Geometry: final body of the model. Coordinates: model frame, mm. Face numbers are marked on the shaded views. A direction names the side the tool comes from. Give positions to 0.01 mm unless a question says otherwise; leave off trailing zeros. Write each loop counter-clockwise with the first axis right and the second up, starting at its lowest first coordinate (ties: lowest second). Pieces come first, ordered by that corner, then holes. Notation, with made-up numbers: (83, 21) - (125, 21) arc R21 cw to (125, 57) - close; hole circle Ø1 at (-34.5, -21). An arc over 180 degrees is marked (long way). Return JSON: item names as keys, results as strings.
from build123d import *

# Parameters (mm, degrees)
SKETCH1_W           = 150
SKETCH1_H           = 150
BASE_FLANGE1_DEPTH  = 7
SKETCH23_W          = 150
SKETCH23_H          = 150
SKETCH23_W_2        = 130
SKETCH23_H_2        = 130
BOSS_EXTRUDE3_DEPTH = 20
SKETCH27_W          = 7
SKETCH27_H          = 150
BOSS_EXTRUDE4_DEPTH = 20
SKETCH28_W          = 150
SKETCH28_H          = 7
BOSS_EXTRUDE5_DEPTH = 20
SKETCH29_W          = 7
SKETCH29_H          = 150
BOSS_EXTRUDE6_DEPTH = 20
SKETCH30_W          = 150
SKETCH30_H          = 7
BOSS_EXTRUDE7_DEPTH = 20
SKETCH31_R          = 2.5
CUT_EXTRUDE1_DEPTH  = 20
SKETCH32_R          = 2.5
CUT_EXTRUDE2_DEPTH  = 20
FILLET1_R           = 5


# Sheet-metal steps are written as plain solids
with BuildPart() as part:
    # Sketch1 → Base-Flange1 (new body)
    with BuildSketch(Plane.XY):
        Rectangle(SKETCH1_W, SKETCH1_H)
    extrude(amount=-BASE_FLANGE1_DEPTH)

    # Sketch23 → Boss-Extrude3 (add)
    with BuildSketch(Plane(origin=(0, 0, -7), x_dir=(-1, 0, 0), z_dir=(0, 0, -1))):
        Rectangle(SKETCH23_W, SKETCH23_H)
        Rectangle(SKETCH23_W_2, SKETCH23_H_2, mode=Mode.SUBTRACT)
    extrude(amount=BOSS_EXTRUDE3_DEPTH)

    # Sketch27 → Boss-Extrude4 (add)
    with BuildSketch(Plane(origin=(75, 0, 0), x_dir=(0, 0, -1), z_dir=(1, 0, 0))):
        with Locations((23.5, 0)):
            Rectangle(SKETCH27_W, SKETCH27_H)
    extrude(amount=BOSS_EXTRUDE4_DEPTH)

    # Sketch28 → Boss-Extrude5 (add)
    with BuildSketch(Plane(origin=(0, -75, 0), x_dir=(-1, 0, 0), z_dir=(0, -1, 0))):
        with Locations((0, 23.5)):
            Rectangle(SKETCH28_W, SKETCH28_H)
    extrude(amount=BOSS_EXTRUDE5_DEPTH)

    # Sketch29 → Boss-Extrude6 (add)
    with BuildSketch(Plane.ZY.offset(75)):
        with Locations((-23.5, 0)):
            Rectangle(SKETCH29_W, SKETCH29_H)
    extrude(amount=BOSS_EXTRUDE6_DEPTH)

    # Sketch30 → Boss-Extrude7 (add)
    with BuildSketch(Plane(origin=(0, 75, 0), x_dir=(1, 0, 0), z_dir=(0, 1, 0))):
        with Locations((0, 23.5)):
            Rectangle(SKETCH30_W, SKETCH30_H)
    extrude(amount=BOSS_EXTRUDE7_DEPTH)

    # Sketch31 → Cut-Extrude1 (cut)
    with BuildSketch(Plane.XY):
        with Locations((-50, -50)):
            Circle(SKETCH31_R)
        with Locations((-50, 50)):
            Circle(SKETCH31_R)
        with Locations((50, 50)):
            Circle(SKETCH31_R)
        with Locations((50, -50)):
            Circle(SKETCH31_R)
        with Locations((37.5, 37.5)):
            Circle(SKETCH31_R)
        with Locations((-37.5, 37.5)):
            Circle(SKETCH31_R)
        with Locations((37.5, -37.5)):
            Circle(SKETCH31_R)
        with Locations((-37.5, -37.5)):
            Circle(SKETCH31_R)
    extrude(amount=-CUT_EXTRUDE1_DEPTH, mode=Mode.SUBTRACT)

    # Sketch32 → Cut-Extrude2 (cut)
    with BuildSketch(Plane.XY.offset(-20)):
        with Locations((85, 55)):
            Circle(SKETCH32_R)
        with Locations((85, -55)):
            Circle(SKETCH32_R)
        with Locations((55, -85)):
            Circle(SKETCH32_R)
        with Locations((-55, -85)):
            Circle(SKETCH32_R)
        with Locations((-85, -55)):
            Circle(SKETCH32_R)
        with Locations((-85, 55)):
            Circle(SKETCH32_R)
        with Locations((-55, 85)):
            Circle(SKETCH32_R)
        with Locations((55, 85)):
            Circle(SKETCH32_R)
    extrude(amount=-CUT_EXTRUDE2_DEPTH, mode=Mode.SUBTRACT)

    # Fillet1
    # the kernel refuses this fillet: 5 mm, written as the material it takes off along each edge
    with BuildSketch(Plane(origin=(70, -70, -5), x_dir=(0, 0, 1), z_dir=(0, -1, 0))) as fillet1_piece_1_section:
        Polygon((0, 0), (FILLET1_R, 0), (FILLET1_R, -FILLET1_R), (0, -FILLET1_R), align=None)
    fillet1_piece_1 = extrude(amount=FILLET1_R, mode=Mode.PRIVATE)
    fillet1_piece_1 = fillet1_piece_1 - Plane(origin=(70, -70, -5), x_dir=(-0.7071067811865475, 0, -0.7071067811865475), z_dir=(0, -1, 0)) * Sphere(FILLET1_R, mode=Mode.PRIVATE)
    add(fillet1_piece_1, mode=Mode.SUBTRACT)
    with BuildSketch(Plane(origin=(70, 70, -5), x_dir=(1, 0, 0), z_dir=(0, 0, 1))) as fillet1_piece_2_section:
        Polygon((0, 0), (FILLET1_R, 0), (FILLET1_R, FILLET1_R), (0, FILLET1_R), align=None)
    fillet1_piece_2 = extrude(amount=FILLET1_R, mode=Mode.PRIVATE)
    fillet1_piece_2 = fillet1_piece_2 - Plane(origin=(70, 70, -5), x_dir=(-0.7071067811865475, -0.7071067811865475, 0), z_dir=(0, 0, 1)) * Sphere(FILLET1_R, mode=Mode.PRIVATE)
    add(fillet1_piece_2, mode=Mode.SUBTRACT)
    with BuildSketch(Plane(origin=(-70, -70, -5), x_dir=(0, 0, 1), z_dir=(0, -1, 0))) as fillet1_piece_3_section:
        Polygon((0, 0), (FILLET1_R, 0), (FILLET1_R, FILLET1_R), (0, FILLET1_R), align=None)
    fillet1_piece_3 = extrude(amount=FILLET1_R, mode=Mode.PRIVATE)
    fillet1_piece_3 = fillet1_piece_3 - Plane(origin=(-70, -70, -5), x_dir=(0.7071067811865475, 0, -0.7071067811865475), z_dir=(0, -1, 0)) * Sphere(FILLET1_R, mode=Mode.PRIVATE)
    add(fillet1_piece_3, mode=Mode.SUBTRACT)
    with BuildSketch(Plane(origin=(-70, 70, -5), x_dir=(-1, 0, 0), z_dir=(0, 0, 1))) as fillet1_piece_4_section:
        Polygon((0, 0), (FILLET1_R, 0), (FILLET1_R, -FILLET1_R), (0, -FILLET1_R), align=None)
    fillet1_piece_4 = extrude(amount=FILLET1_R, mode=Mode.PRIVATE)
    fillet1_piece_4 = fillet1_piece_4 - Plane(origin=(-70, 70, -5), x_dir=(0.7071067811865475, -0.7071067811865475, 0), z_dir=(0, 0, 1)) * Sphere(FILLET1_R, mode=Mode.PRIVATE)
    add(fillet1_piece_4, mode=Mode.SUBTRACT)
    with BuildSketch(Plane(origin=(75, -75, -20), x_dir=(-1, 0, 0), z_dir=(0, 0, 1)), Plane(origin=(75, 75, -20), x_dir=(0, -1, 0), z_dir=(0, 0, 1)), Plane(origin=(-75, -75, -5), x_dir=(1, 0, 0), z_dir=(0, 0, -1)), Plane(origin=(-75, 75, -5), x_dir=(0, -1, 0), z_dir=(0, 0, -1))) as fillet1_piece_5:
        with BuildLine():
            CenterArc((FILLET1_R, -FILLET1_R), FILLET1_R, 90, 90)
            Line((0, -FILLET1_R), (0, 0))
            Line((0, 0), (FILLET1_R, 0))
        make_face()
    extrude(amount=15, mode=Mode.SUBTRACT)
    with BuildSketch(Plane(origin=(-70, -75, 0), x_dir=(0, 0, -1), z_dir=(1, 0, 0))) as fillet1_piece_6:
        with BuildLine():
            CenterArc((FILLET1_R, FILLET1_R), FILLET1_R, 180, 90)
            Line((0, FILLET1_R), (0, 0))
            Line((0, 0), (FILLET1_R, 0))
        make_face()
    extrude(amount=140, mode=Mode.SUBTRACT)
    with BuildSketch(Plane(origin=(-75, 70, 0), x_dir=(1, 0, 0), z_dir=(0, -1, 0)), Plane(origin=(70, 75, 0), x_dir=(0, -1, 0), z_dir=(-1, 0, 0)), Plane(origin=(75, -70, 0), x_dir=(-1, 0, 0), z_dir=(0, 1, 0))) as fillet1_piece_7:
        with BuildLine():
            CenterArc((FILLET1_R, -FILLET1_R), FILLET1_R, 90, 90)
            Line((0, -FILLET1_R), (0, 0))
            Line((0, 0), (FILLET1_R, 0))
        make_face()
    extrude(amount=140, mode=Mode.SUBTRACT)


solid = part.part
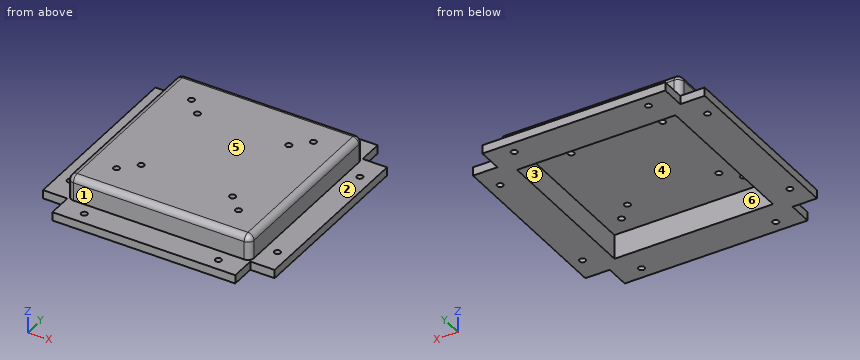
Q1. Mould query, pull axis X, two halves, no side actions, for the marked faces 4, 5 and 6. Classes: pulls with the +X half, pulls with the -X half, needs draft (parallel to the pull), parting line crosses it, or undercut.
Answer key:
{"face 4": "undercut", "face 5": "needs draft", "face 6": "undercut"}
Q2. Section query D-D, the plane y = -55. Return the cut outline in (x, z).
Answer key:
{"outline": "(-95, -27) - (-87.5, -27) - (-87.5, -20) - (-95, -20) - close; (-82.5, -27) - (-65, -27) - (-65, -7) - (65, -7) - (65, -27) - (82.5, -27) - (82.5, -20) - (75, -20) - (75, -5) arc R5 ccw to (70, 0) - (-70, 0) arc R5 ccw to (-75, -5) - (-75, -20) - (-82.5, -20) - close; (87.5, -27) - (95, -27) - (95, -20) - (87.5, -20) - close"}
Q3. Set-up query: the marked faces 1, 2 and 3. Return all of +Z, -Z, +X, -X, +Y, -Y with unobstructed straight access to the full face (end or side cutting, diameter ignored); none if empty.
Answer key:
{"face 1": "+Z, +X, -X, -Y", "face 2": "+Z", "face 3": "-Z"}
Q4. Material intervals for probe 1 along Y at (x, z) = (-85, -24.5); probe 2 along Y at (x, z) = (50, -4.5); probe 3 along X at (y, z) = (-37, -16.75), sorted ascending. Write a range as [from, to].
Answer key:
{"probe 1": "y = [-75, -57.5], [-52.5, 52.5], [57.5, 75]", "probe 2": "y = [-74.97, -52.5], [-47.5, 47.5], [52.5, 74.97]", "probe 3": "x = [-75, -65], [65, 75]"}
Q5. Section query C-C, the plane z = -24. Count the separate pieces of the cut face and the enclosed holes in it, plus the area to 3 significant figures.
Answer key:
{"separate pieces": "1", "enclosed holes": "9", "area": "17,400 mm^2"}
Q6. Pin query (flat end, axial travel): P1, Ø3.5, axis at x = 86.5, z = -22, coming from the -Y side; P2, Ø3, axis at y = -53, z = -5.5, coming from the +X side; P3, Ø8, axis at x = 37.5, y = 37.5, coming from the -Z side; P4, Ø3, axis at x = 85, y = -55, coming from the -Z side. Return the tip coordinate at first contact, or that it passes through.
Answer key:
{"P1": "stops at y = -75", "P2": "stops at x = 75", "P3": "stops at z = -7", "P4": "passes through"}
Q7. Section query A-A, the plane x = 85. Return the cut outline in (y, z).
Answer key:
{"outline": "(-75, -27) - (-57.5, -27) - (-57.5, -20) - (-75, -20) - close; (-52.5, -27) - (52.5, -27) - (52.5, -20) - (-52.5, -20) - close; (57.5, -27) - (75, -27) - (75, -20) - (57.5, -20) - close"}
